Part model, mm, in its own coordinate system. A direction names the side the tool comes from. Give positions to 0.01 mm unless a question says otherwise; leave off trailing zeros. Order: outer loops, then holes, each group sorted by start corner. A loop starts at its lowest first (then second) coordinate and runs counter-clockwise, first axis right, second up. Notation, with made-up numbers: (-0.5, 81) - (6.5, 81) arc R16 ccw to (6.5, 111) - close; hole circle Ø4 at (-27, 39.25). An arc over 180 degrees is marked (long way). One line per item, written item: value.
```python
from build123d import *

# Parameters (mm, degrees)
F1_DEPTH = 25.4
F2_R     = 6.35
F3_R     = 3.17499
F4_R     = 9.525
F5_DEPTH = 152.401


# Not quite as in the source:
# - a fillet or chamfer is up to 0.001 mm smaller than in the source, because OpenCascade refuses the exact size


with BuildPart() as f1:
    # F0 (on Front) → F1 (new body, symmetric)
    with BuildSketch(Plane.XZ):
        Polygon((-76.2, 0), (0, 0), (76.2, 0), (76.2, 50.8), (69.85, 50.8), (69.85, 6.35), (0, 6.35), (-69.85, 6.35), (-69.85, 50.8), (-76.2, 50.8), align=None)
    extrude(amount=F1_DEPTH, both=True)

    # F2
    f2_edges = [f1.edges().sort_by_distance(p)[0] for p in [
        (-69.85, 0, 6.35),
        (69.85, 0, 6.35),
        (76.2, 0, 0),
        (-76.2, 0, 0),
    ]]
    fillet(f2_edges, radius=F2_R)

    # F3 (radius 3.175 in the source; OpenCascade refuses exactly that, so slightly less here)
    f3_edges = [f1.edges().sort_by_distance(p)[0] for p in [
        (-69.85, 0, 50.8),
        (-76.2, 0, 50.8),
        (69.85, 0, 50.8),
        (76.2, 0, 50.8),
    ]]
    fillet(f3_edges, radius=F3_R)

    # F4 (on face) → F5 (cut, through all)
    with BuildSketch(Plane(origin=(-76.2, 0, 0), x_dir=(0, -1, 0), z_dir=(-1, 0, 0))):
        with Locations((0, 35.2541096509)):
            Circle(F4_R)
    extrude(amount=-F5_DEPTH, mode=Mode.SUBTRACT)


solid = f1.part
```
1) Two-plate mould, pull along X, no slides. Class faces 1 (the face through (-70.8, 0.36, 49.89)), 2 (the face through (-1, 0, 0)), 3 (the face through (70.8, -0.36, 49.89)), 4 (the face through (75.29, -0.36, 49.85)): pulls with the +X half, pulls with the -X half, needs draft (parallel to the pull), parting line crosses it, or undercut.
Answer:
face 1: undercut
face 2: needs draft
face 3: undercut
face 4: pulls with the +X half
2) Slice it at A-A on z = 22. Write the cut outline in (x, y).
Answer:
outline: (-76.2, -25.4) - (-69.85, -25.4) - (-69.85, 25.4) - (-76.2, 25.4) - close; (69.85, -25.4) - (76.2, -25.4) - (76.2, 25.4) - (69.85, 25.4) - close
3) Which spindle directions (+Z, -Z, +X, -X, +Y, -Y) get a long thin tool onto all of the face, cutting with end or side? Do faces 5 (the face through (0, 25.4, 5)), 6 (the face through (-69.85, -6, 26)). Say none if no direction does.
Answer:
face 5: +Z, -Z, +X, -X, +Y
face 6: +Z, +Y, -Y
4) Slice it at C-C on z = 33. Write the cut outline in (x, y).
Answer:
outline: (-76.2, -25.4) - (-69.85, -25.4) - (-69.85, -9.25) - (-76.2, -9.25) - close; (-76.2, 9.25) - (-69.85, 9.25) - (-69.85, 25.4) - (-76.2, 25.4) - close; (69.85, -25.4) - (76.2, -25.4) - (76.2, -9.25) - (69.85, -9.25) - close; (69.85, 9.25) - (76.2, 9.25) - (76.2, 25.4) - (69.85, 25.4) - close
5) Wall check: line 1 along X through (y, z) = (-12, 20); line 2 along X through (y, z) = (-8, 6). Give the ranges that are in metal, low to high. Write a range as [from, to].
Answer:
line 1: x = [-76.2, -69.85], [69.85, 76.2]
line 2: x = [-76.19, 76.19]
6) Drop a flat-ended pin along its axis: P1, Ø2, axis at x = -23, y = -9.5, coming from the +Z side. Give the stop position or say it passes through.
Answer:
P1: stops at z = 6.35
7) Slice it at B-B on y = 0. Count the separate pieces of the cut face and the enclosed holes in it, then the cut area to 3 significant figures.
Answer:
separate pieces: 3
enclosed holes: 0
area: 1,280 mm2
